from build123d import *

# Parameters (mm, degrees)
BOSS_EXTRU_1_DEPTH = 1
ESQUISSE2_R        = 16
BOSS_EXTRU_2_DEPTH = 55
ESQUISSE3_R        = 17
BOSS_EXTRU_3_DEPTH = 20
CONG_1_R           = 15
CONG_2_R           = 0.5
ESQUISSE4_R        = 3
BOSS_EXTRU_4_DEPTH = 8


with BuildPart() as part:
    # Esquisse1 → Boss.-Extru.1 (new body)
    with BuildSketch(Plane(origin=(0, 0, 0), x_dir=(1, 0, 0), z_dir=(0, 1, 0))):
        with BuildLine():
            Line((2, 0), (42, 0))
            ThreePointArc((42, 0), (43.414213562, 0.585786438), (44, 2))
            Line((44, 2), (44, 32))
            ThreePointArc((44, 32), (43.414213562, 33.414213562), (42, 34))
            Line((42, 34), (2, 34))
            ThreePointArc((2, 34), (0.585786438, 33.414213562), (0, 32))
            Line((0, 32), (0, 2))
            ThreePointArc((0, 2), (0.585786438, 0.585786438), (2, 0))
        make_face()
    extrude(amount=BOSS_EXTRU_1_DEPTH)

    # Esquisse2 → Boss.-Extru.2 (add)
    with BuildSketch(Plane.XZ):
        with Locations(Location((22, -17, 0), (0, 0, 270))):
            Circle(ESQUISSE2_R)
    extrude(amount=BOSS_EXTRU_2_DEPTH)

    # Esquisse3 → Boss.-Extru.3 (add)
    with BuildSketch(Plane.XZ.offset(55)):
        with Locations(Location((22, -17, 0), (0, 0, 270))):
            Circle(ESQUISSE3_R)
    extrude(amount=BOSS_EXTRU_3_DEPTH)

    # Congé1
    cong_1_edges = [part.edges().sort_by_distance(p)[0] for p in [
        (22, -75, 0),
    ]]
    fillet(cong_1_edges, radius=CONG_1_R)

    # Congé2
    cong_2_edges = [part.edges().sort_by_distance(p)[0] for p in [
        (22, -55, 0),
    ]]
    fillet(cong_2_edges, radius=CONG_2_R)

    # Esquisse4 → Boss.-Extru.4 (add)
    with BuildSketch(Plane(origin=(0, 1, 0), x_dir=(1, 0, 0), z_dir=(0, 1, 0))):
        with Locations(Location((22, 17, 0), (0, 0, 90))):
            Circle(ESQUISSE4_R)
    extrude(amount=BOSS_EXTRU_4_DEPTH)


solid = part.part
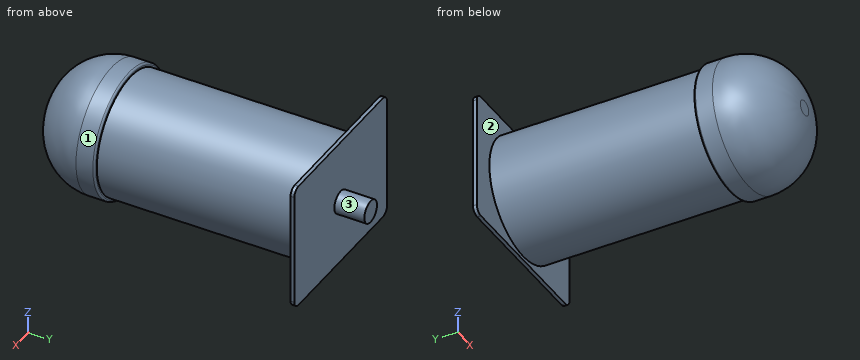
Design review of the part built by this model. Coordinates are the model's own, in mm. Face numbers are marked on the shaded views. A direction names the side the tool comes from. Round coordinates to 2 decimals unless told otherwise and drop trailing zeros. Write each loop counter-clockwise with the first axis right and the second up, starting at its lowest first coordinate (ties: lowest second). Pieces come first, ordered by that corner, then holes. Notation, with made-up numbers: (60, 21.5) - (97, 21.5) arc R24 cw to (97, 53.5) - close; hole circle Ø10 at (18.25, 20.5). An arc over 180 degrees is marked (long way). Return JSON: item names as keys, results as strings. Group by question number.
Item 1: We need section B-B on y = -44.5. Write out the cut boundary in (x, z).
Item 2: Machinability: for the marked faces 1, 2 and 3, which of the approach directions +Z, -Z, +X, -X, +Y, -Y give a long, thin tool a straight path to every point of the face, cutting with its end or side? Answer none if there is none.
Item 3: Insertion check: P1, Ø12, axis at x = 10.5, y = -39.5, coming from the -Z side (3 decimals); P2, Ø1, axis at x = 32.5, y = -48, coming from the +Z side; P3, Ø8, axis at x = 19, y = -48.5, coming from the -Z side. Each pin has a flat end and moves straight along its axis. Give the tip position at first contact, or say it passes through.
Item 4: We need section A-A on x = 3.5. Write out the cut boundary in (y, z), and give its area (3 significant figures).
Item 5: For probe 1 along Y at (x, z) = (35.5, -31.5); probe 2 along Y at (x, z) = (32.5, -29.5); probe 3 along X at (y, z) = (-54, -17.5), list the stretches that pass through material, from the lowest coordinate up. Write a range as [from, to].
Model answer:
{
 "1": {"outline": "circle Ø32 at (22, -17)"},
 "2": {"face 1": "-Y", "face 2": "none", "face 3": "+Y"},
 "3": {"P1": "stops at z = -32.025", "P2": "stops at z = -4.51", "P3": "stops at z = -33"},
 "4": {"outline": "(0, -34) - (1, -34) - (1, 0) - (0, 0) - close", "area": "34.0 mm²"},
 "5": {"probe 1": "y = [0, 1]", "probe 2": "y = [-64.45, -55], [0, 1]", "probe 3": "x = [6.01, 37.99]"}
}
